from build123d import *

# Parameters (mm, degrees)
F0_W     = 56
F0_H     = 56
F1_DEPTH = 0.5
F2_R     = 4


with BuildPart() as f1:
    # F0 (on Top) → F1 (new body)
    with BuildSketch(Plane.XY):
        with BuildLine():
            Line((27.535898, 33), (-27.535898, 33))
            ThreePointArc((-27.535898, 33), (-27.136297, 32.035276), (-27, 31))
            ThreePointArc((-27, 31), (-29, 27.535898), (-33, 27.535898))
            Line((-33, 27.535898), (-33, -27.535898))
            ThreePointArc((-33, -27.535898), (-29, -27.535898), (-27, -31))
            ThreePointArc((-27, -31), (-27.136297, -32.035276), (-27.535898, -33))
            Line((-27.535898, -33), (27.535898, -33))
            ThreePointArc((27.535898, -33), (28.171573, -28.171573), (33, -27.535898))
            Line((33, -27.535898), (33, 27.535898))
            ThreePointArc((33, 27.535898), (28.171573, 28.171573), (27.535898, 33))
        make_face()
        Rectangle(F0_W, F0_H, mode=Mode.SUBTRACT)
        with BuildLine():
            Line((31, 35), (-31, 35))
            ThreePointArc((-31, 35), (-29, 34.464102), (-27.535898, 33))
            Line((-27.535898, 33), (27.535898, 33))
            ThreePointArc((27.535898, 33), (29, 34.464102), (31, 35))
        make_face()
        with BuildLine():
            ThreePointArc((35, 31), (33.828427, 33.828427), (31, 35))
            ThreePointArc((31, 35), (29, 34.464102), (27.535898, 33))
            ThreePointArc((27.535898, 33), (28.171573, 28.171573), (33, 27.535898))
            ThreePointArc((33, 27.535898), (34.464102, 29), (35, 31))
        make_face()
        with BuildLine():
            Line((35, -31), (35, 31))
            ThreePointArc((35, 31), (34.464102, 29), (33, 27.535898))
            Line((33, 27.535898), (33, -27.535898))
            ThreePointArc((33, -27.535898), (34.464102, -29), (35, -31))
        make_face()
        with BuildLine():
            ThreePointArc((31, -35), (33.828427, -33.828427), (35, -31))
            ThreePointArc((35, -31), (34.464102, -29), (33, -27.535898))
            ThreePointArc((33, -27.535898), (28.171573, -28.171573), (27.535898, -33))
            ThreePointArc((27.535898, -33), (29, -34.464102), (31, -35))
        make_face()
        with BuildLine():
            ThreePointArc((-27.535898, -33), (-29, -34.464102), (-31, -35))
            Line((-31, -35), (31, -35))
            ThreePointArc((31, -35), (29, -34.464102), (27.535898, -33))
            Line((27.535898, -33), (-27.535898, -33))
        make_face()
        with BuildLine():
            ThreePointArc((-33, 27.535898), (-34.464102, 29), (-35, 31))
            Line((-35, 31), (-35, -31))
            ThreePointArc((-35, -31), (-34.464102, -29), (-33, -27.535898))
            Line((-33, -27.535898), (-33, 27.535898))
        make_face()
        with BuildLine():
            ThreePointArc((-33, -27.535898), (-34.464102, -29), (-35, -31))
            ThreePointArc((-35, -31), (-33.828427, -33.828427), (-31, -35))
            ThreePointArc((-31, -35), (-29, -34.464102), (-27.535898, -33))
            ThreePointArc((-27.535898, -33), (-27.136297, -32.035276), (-27, -31))
            ThreePointArc((-27, -31), (-29, -27.535898), (-33, -27.535898))
        make_face()
        with BuildLine():
            ThreePointArc((-27.535898, 33), (-29, 34.464102), (-31, 35))
            ThreePointArc((-31, 35), (-33.828427, 33.828427), (-35, 31))
            ThreePointArc((-35, 31), (-34.464102, 29), (-33, 27.535898))
            ThreePointArc((-33, 27.535898), (-29, 27.535898), (-27, 31))
            ThreePointArc((-27, 31), (-27.136297, 32.035276), (-27.535898, 33))
        make_face()
    extrude(amount=-F1_DEPTH)

    # F2
    f2_edges = [f1.edges().sort_by_distance(p)[0] for p in [
        (-28, -28, -0.25),
        (-28, 28, -0.25),
        (28, 28, -0.25),
        (28, -28, -0.25),
    ]]
    fillet(f2_edges, radius=F2_R)


solid = f1.part
Work out the finished part from the listing and answer in its coordinate system (mm). A direction names the side the tool comes from. Give positions to 0.01 mm unless a question says otherwise; leave off trailing zeros. Order: outer loops, then holes, each group sorted by start corner. A loop starts at its lowest first (then second) coordinate and runs counter-clockwise, first axis right, second up. Notation, with made-up numbers: (-8.5, -1.5) -> (9.5, -1.5) arc R19 cw to (9.5, 31.5) -> close; hole circle Ø11 at (0.5, 36.5). An arc over 180 degrees is marked (long way). Answer as a JSON object with one key per item and string values. Group by question number.
1. Consider line 1 along X through (y, z) = (17.5, -0.25); line 2 along Y through (x, z) = (-25.5, -0.05). Determine where each line is inside the solid, lowest interval first. Write a range as [from, to].
2. A tool of negligible diameter and unlimited length cuts with its end or side. For faces 1 (the cylindrical face through (-26.859, 26.797, -0.254)), 2 (the flat face through (-32, 0, -0.5)), from which of +Z, -Z, +X, -X, +Y, -Y can it reach the whole face along a straight path? Write none if from no direction.
3. The mould has two halves that part along X. Classify faces 3 (the flat face through (-32, 0, 0)), 4 (the cylindrical face through (33.859, 33.797, -0.246)), 5 (the cylindrical face through (-33.797, 33.859, -0.246)), 6 (the cylindrical face through (26.797, -26.859, -0.254)): released by +X, released by -X, zero draft, split by the parting line, or undercut.
4. Section A-A on y = -7 is taken. Determine the outline of the cut face in (x, z), plus the area to 3 significant figures.
5. Section C-C on z = -0.35 is taken. Determine the outline of the cut face in (x, y), plus the area to 3 significant figures.
Result sheet:
{
 "1": {"line 1": "x = [-35, -28], [28, 35]", "line 2": "y = [-35, -27.71], [27.71, 35]"},
 "2": {"face 1": "+Z, -Z", "face 2": "-Z, +X, -X, +Y, -Y"},
 "3": {"face 3": "zero draft", "face 4": "released by +X", "face 5": "released by -X", "face 6": "undercut"},
 "4": {"outline": "(-35, -0.5) -> (-28, -0.5) -> (-28, 0) -> (-35, 0) -> close; (28, -0.5) -> (35, -0.5) -> (35, 0) -> (28, 0) -> close", "area": "7.00 mm^2"},
 "5": {"outline": "(-35, -31) arc R4 ccw to (-31, -35) -> (31, -35) arc R4 ccw to (35, -31) -> (35, 31) arc R4 ccw to (31, 35) -> (-31, 35) arc R4 ccw to (-35, 31) -> close; hole (-28, -24) arc R4 ccw to (-24, -28) -> (24, -28) arc R4 ccw to (28, -24) -> (28, 24) arc R4 ccw to (24, 28) -> (-24, 28) arc R4 ccw to (-28, 24) -> close", "area": "1,760 mm^2"}
}
